from build123d import *

# Parameters (mm, degrees)
SKETCH1_R                = 37.5
BOSS_EXTRUDE1_DEPTH      = 47.25
BOSS_EXTRUDE2_DEPTH      = 41.55
BOSS_EXTRUDE2_DEPTH_BACK = 39.70459341
SKETCH2_R                = 37.5
CUT_EXTRUDE1_DEPTH       = 74.247627948
CUT_EXTRUDE1_DEPTH_BACK  = 74.247627948
SKETCH4_R                = 6
BOSS_EXTRUDE3_DEPTH      = 60
SKETCH5_R                = 7.5
BOSS_EXTRUDE4_DEPTH      = 5.85
CUT_EXTRUDE2_DEPTH       = 140.682215941
CUT_EXTRUDE2_DEPTH_BACK  = 58.15
SKETCH6_R                = 6


with BuildPart() as part:
    # Sketch1 → Boss-Extrude1 (new body)
    with BuildSketch(Plane(origin=(0, 0, 0), x_dir=(0, 0, -1), z_dir=(1, 0, 0))):
        Circle(SKETCH1_R)
    extrude(amount=BOSS_EXTRUDE1_DEPTH)

    # Sketch2 → Boss-Extrude2 (add, two sides: drawn at the far end of the back side and taken through both)
    with BuildSketch(Plane(origin=(0, 0, 0), x_dir=(1, 0, 0), z_dir=(0, 1, 0)).offset(-BOSS_EXTRUDE2_DEPTH_BACK)):
        with Locations(Location((0, 0, 0), (0, 0, 270))):
            Circle(SKETCH2_R)
    extrude(amount=BOSS_EXTRUDE2_DEPTH + BOSS_EXTRUDE2_DEPTH_BACK)

    # Sketch3 → Cut-Extrude1 (cut, two sides: drawn at the far end of the back side and taken through both)
    with BuildSketch(Plane.XY.offset(-CUT_EXTRUDE1_DEPTH_BACK)):
        Polygon((37.5, -39.70459341), (-37.5, -39.70459341), (-37.5, -9.70456466), align=None)
    extrude(amount=CUT_EXTRUDE1_DEPTH + CUT_EXTRUDE1_DEPTH_BACK, mode=Mode.SUBTRACT)

    # Sketch4 → Boss-Extrude3 (add)
    with BuildSketch(Plane(origin=(47.25, 0, 0), x_dir=(0, 0, -1), z_dir=(1, 0, 0))):
        Circle(SKETCH4_R)
    extrude(amount=BOSS_EXTRUDE3_DEPTH)

    # Sketch5 → Boss-Extrude4 (add)
    with BuildSketch(Plane(origin=(47.25, 0, 0), x_dir=(0, 0, -1), z_dir=(1, 0, 0))):
        Circle(SKETCH5_R)
    extrude(amount=BOSS_EXTRUDE4_DEPTH)

    # Sketch6 → Cut-Extrude2 (cut, two sides: drawn at the far end of the back side and taken through both)
    with BuildSketch(Plane(origin=(0, 41.55, 0), x_dir=(1, 0, 0), z_dir=(0, 1, 0)).offset(-CUT_EXTRUDE2_DEPTH_BACK)):
        with Locations(Location((0, 0, 0), (0, 0, 90))):
            Circle(SKETCH6_R)
    extrude(amount=CUT_EXTRUDE2_DEPTH + CUT_EXTRUDE2_DEPTH_BACK, mode=Mode.SUBTRACT)


solid = part.part
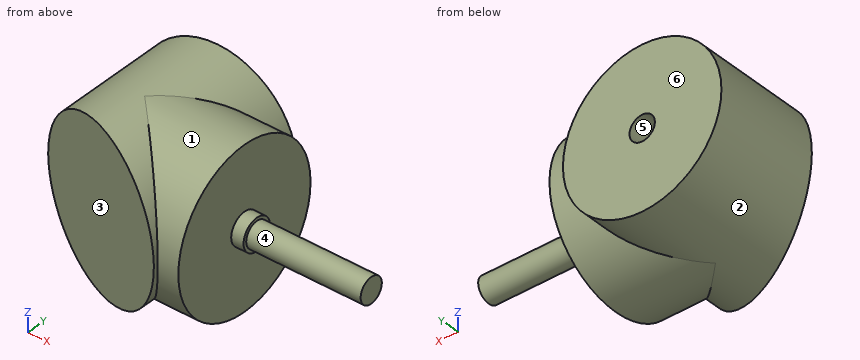
For this review, take the finished solid that the model builds, in its own axes (mm). Face numbers are marked on the shaded views. A direction names the side the tool comes from. Round coordinates to 2 decimals unless told otherwise and drop trailing zeros. Loops run counter-clockwise (first coordinate to the right, second up) from the corner with the lowest first, then second, coordinate; pieces in that order, holes last. Notation, with made-up numbers: (69.5, -25.5) - (81.5, -25.5) arc R22 ccw to (81.5, 11.5) - close; hole circle Ø5 at (-26.5, 22). An arc over 180 degrees is marked (long way). Put each result on its own line as item: value. Start each with the question number.
1. Insertion check: P1, Ø1.5, axis at x = 23.5, z = -1, coming from the -Y side; P2, Ø19, axis at x = 0, z = 0, coming from the -Y side; P3, Ø2, axis at y = 18, z = -13, coming from the -X side. Each pin has a flat end and moves straight along its axis. Give the tip position at first contact, or say it passes through.
2. Mouldability with a two-part tool opening along Z and no side actions: class the marked faces 4, 5 and 6 as +Z half, -Z half, draft (parallel to the pull), parting line (faces both ways), or undercut.
3. Consider section D-D on y = -29.5. State the section outline as (x, z) points.
4. Consider section C-C on x = 1.5. State the section outline as (y, z) points, plus the area to 3 significant figures.
5. Consider section A-A on y = 0. State the section outline as (x, z) points.
6. Consider section B-B on z = 0. State the section outline as (x, y) points.
7. For probe 1 along X at (y, z) = (24.5, 0); probe 2 along X at (y, z) = (-2, 0); probe 3 along Y at (x, z) = (27, -33), list the stretches that pass through material, from the lowest coordinate up. Write a range as [from, to].
8. For the marked faces 1, 2 and 3, list the 3-axis set-ups (+Z, -Z, +X, -X, +Y, -Y) from which the entire face can be reached by the end or side of a thin tool; tool diameter is ignored.
Result sheet:
1. P1: y = -34.4
1. P2: y = -28.5
1. P3: x = -35.53
2. face 4: parting line
2. face 5: undercut
2. face 6: draft
3. outline: (11.99, -35.53) arc R37.5 ccw to (29.5, -23.15) - (47.25, -23.15) - (47.25, 23.15) - (29.5, 23.15) arc R37.5 ccw to (11.99, 35.53) - close
4. outline: (-25.3, -37.47) - (-1.5, -37.47) arc R37.5 ccw to (1.5, -37.47) - (41.55, -37.47) - (41.55, -5.81) - (-16.6, -5.81) - (-16.6, 5.81) - (41.55, 5.81) - (41.55, 37.47) - (1.5, 37.47) arc R37.5 ccw to (-1.5, 37.47) - (-25.3, 37.47) - close
4. area: 4,330 mm^2
5. outline: (0, -37.5) - (47.25, -37.5) - (47.25, -7.5) - (53.1, -7.5) - (53.1, -6) - (107.25, -6) - (107.25, 6) - (53.1, 6) - (53.1, 7.5) - (47.25, 7.5) - (47.25, 37.5) - (0, 37.5) arc R37.5 ccw to start; hole circle Ø12 at (0, 0)
6. outline: (-37.5, -9.7) - (37.5, -39.7) - (37.5, -37.5) - (47.25, -37.5) - (47.25, -7.5) - (53.1, -7.5) - (53.1, -6) - (107.25, -6) - (107.25, 6) - (53.1, 6) - (53.1, 7.5) - (47.25, 7.5) - (47.25, 37.5) - (37.5, 37.5) - (37.5, 41.55) - (6, 41.55) - (6, -16.6) - (-6, -16.6) - (-6, 41.55) - (-37.5, 41.55) - close
7. probe 1: [-37.5, -6], [6, 47.25]
7. probe 2: [-37.5, -6], [6, 107.25]
7. probe 3: [-17.81, 17.81]
8. face 1: +X
8. face 2: none
8. face 3: +Z, -Z, -X, -Y
